Build history of the part. All positions in model axes, mm. Face numbers are marked on the shaded views. Round coordinates to 2 decimals unless told otherwise and drop trailing zeros. One line per item, written item: value. Start each with the question number.
Item 1: Pin check, flat tips, straight feed: pin 1 (3.5 mm diameter, centred on x = 11.5, z = 5, fed in from -Y); pin 2 (4 mm diameter, centred on x = 7.5, z = 0, fed in from -Y); pin 3 (2.5 mm diameter, centred on x = 11.96, z = 11.94, fed in from -Y). Stop position of each tip, or through.
Item 2: Band-saw the part on A-A, the plane y = -2.1. Give the number of separate pieces and of enclosed holes in the cut face, then the cut area to 3 significant figures.
Item 3: Probe L1, parallel to Z at x = -20.5, y = -1.85 (3 decimals); L2, parallel to X at y = -2.75, z = 5.5 (3 decimals); L3, parallel to Z at x = 13, y = -0.75 (3 decimals). List the from-to ranges inside material, lowest first.
Item 4: Two-plate mould, pull along Z, no slides. Class the marked faces 1 and 2: +Z half, -Z half, draft (parallel to the pull), parting line (faces both ways), or undercut.
```python
from build123d import *

# Parameters (mm, degrees)
SKETCH1_W           = 47.81
SKETCH1_H           = 31.85
BOSS_EXTRUDE1_DEPTH = 3.16
SKETCH2_R           = 2.445
BOSS_EXTRUDE2_DEPTH = 1.7
SHELL1_T            = -0.78
SKETCH3_R           = 2.35
SKETCH3_R_2         = 2.175
BOSS_EXTRUDE3_DEPTH = 2.18


with BuildPart() as part:
    # Sketch1 → Boss-Extrude1 (new body)
    with BuildSketch(Plane(origin=(0, 0, 0), x_dir=(1, 0, 0), z_dir=(0, 1, 0))):
        Rectangle(SKETCH1_W, SKETCH1_H)
    extrude(amount=-BOSS_EXTRUDE1_DEPTH)

    # Sketch2 → Boss-Extrude2 (add)
    with BuildSketch(Plane(origin=(0, 0, 0), x_dir=(1, 0, 0), z_dir=(0, 1, 0))):
        with Locations(Location((19.920833333, 11.94375, 0), (0, 0, 270))):
            Circle(SKETCH2_R)
        with Locations(Location((11.960833333, 11.94375, 0), (0, 0, 270))):
            Circle(SKETCH2_R)
        with Locations(Location((4.000833333, 11.94375, 0), (0, 0, 270))):
            Circle(SKETCH2_R)
        with Locations(Location((-3.959166667, 11.94375, 0), (0, 0, 270))):
            Circle(SKETCH2_R)
        with Locations(Location((-11.919166667, 11.94375, 0), (0, 0, 270))):
            Circle(SKETCH2_R)
        with Locations(Location((-19.879166667, 11.94375, 0), (0, 0, 270))):
            Circle(SKETCH2_R)
        with Locations(Location((11.960833333, 3.98375, 0), (0, 0, 270))):
            Circle(SKETCH2_R)
        with Locations(Location((4.000833333, 3.98375, 0), (0, 0, 270))):
            Circle(SKETCH2_R)
        with Locations(Location((-3.959166667, 3.98375, 0), (0, 0, 270))):
            Circle(SKETCH2_R)
        with Locations(Location((-11.919166667, 3.98375, 0), (0, 0, 270))):
            Circle(SKETCH2_R)
        with Locations(Location((-19.879166667, 3.98375, 0), (0, 0, 270))):
            Circle(SKETCH2_R)
        with Locations(Location((11.960833333, -3.97625, 0), (0, 0, 270))):
            Circle(SKETCH2_R)
        with Locations(Location((4.000833333, -3.97625, 0), (0, 0, 270))):
            Circle(SKETCH2_R)
        with Locations(Location((-3.959166667, -3.97625, 0), (0, 0, 270))):
            Circle(SKETCH2_R)
        with Locations(Location((-11.919166667, -3.97625, 0), (0, 0, 270))):
            Circle(SKETCH2_R)
        with Locations(Location((-19.879166667, -3.97625, 0), (0, 0, 270))):
            Circle(SKETCH2_R)
        with Locations(Location((11.960833333, -11.93625, 0), (0, 0, 270))):
            Circle(SKETCH2_R)
        with Locations(Location((4.000833333, -11.93625, 0), (0, 0, 270))):
            Circle(SKETCH2_R)
        with Locations(Location((-3.959166667, -11.93625, 0), (0, 0, 270))):
            Circle(SKETCH2_R)
        with Locations(Location((-11.919166667, -11.93625, 0), (0, 0, 270))):
            Circle(SKETCH2_R)
        with Locations(Location((-19.879166667, -11.93625, 0), (0, 0, 270))):
            Circle(SKETCH2_R)
        with Locations(Location((19.920833333, 3.98375, 0), (0, 0, 270))):
            Circle(SKETCH2_R)
        with Locations(Location((19.920833333, -3.97625, 0), (0, 0, 270))):
            Circle(SKETCH2_R)
        with Locations(Location((19.920833333, -11.93625, 0), (0, 0, 270))):
            Circle(SKETCH2_R)
    extrude(amount=BOSS_EXTRUDE2_DEPTH)

    # Shell1
    shell1_openings = [part.faces().sort_by_distance(p)[0] for p in [
        (0, -3.16, 0),
    ]]
    offset(amount=SHELL1_T, openings=shell1_openings, kind=Kind.INTERSECTION)

    # Sketch3 → Boss-Extrude3 (add)
    # profile 1 of 15: a face of its own
    with BuildSketch(Plane.XZ.offset(0.78)):
        with Locations(Location((-15.936666667, 7.9625, 0), (0, 0, 90))):
            Circle(SKETCH3_R)
        with Locations(Location((-15.936666667, 7.9625, 0), (0, 0, 90))):
            Circle(SKETCH3_R_2, mode=Mode.SUBTRACT)
    # profile 2 of 15: a face of its own
    with BuildSketch(Plane.XZ.offset(0.78)):
        with Locations(Location((-7.966666667, 7.9625, 0), (0, 0, 90))):
            Circle(SKETCH3_R)
        with Locations(Location((-7.966666667, 7.9625, 0), (0, 0, 90))):
            Circle(SKETCH3_R_2, mode=Mode.SUBTRACT)
    # profile 3 of 15: a face of its own
    with BuildSketch(Plane.XZ.offset(0.78)):
        with Locations(Location((0.003333333, 7.9625, 0), (0, 0, 90))):
            Circle(SKETCH3_R)
        with Locations(Location((0.003333333, 7.9625, 0), (0, 0, 90))):
            Circle(SKETCH3_R_2, mode=Mode.SUBTRACT)
    # profile 4 of 15: a face of its own
    with BuildSketch(Plane.XZ.offset(0.78)):
        with Locations(Location((7.973333333, 7.9625, 0), (0, 0, 90))):
            Circle(SKETCH3_R)
        with Locations(Location((7.973333333, 7.9625, 0), (0, 0, 90))):
            Circle(SKETCH3_R_2, mode=Mode.SUBTRACT)
    # profile 5 of 15: a face of its own
    with BuildSketch(Plane.XZ.offset(0.78)):
        with Locations(Location((15.943333333, 7.9625, 0), (0, 0, 90))):
            Circle(SKETCH3_R)
        with Locations(Location((15.943333333, 7.9625, 0), (0, 0, 90))):
            Circle(SKETCH3_R_2, mode=Mode.SUBTRACT)
    # profile 6 of 15: a face of its own
    with BuildSketch(Plane.XZ.offset(0.78)):
        with Locations(Location((-7.966666667, 0.0025, 0), (0, 0, 90))):
            Circle(SKETCH3_R)
        with Locations(Location((-7.966666667, 0.0025, 0), (0, 0, 90))):
            Circle(SKETCH3_R_2, mode=Mode.SUBTRACT)
    # profile 7 of 15: a face of its own
    with BuildSketch(Plane.XZ.offset(0.78)):
        with Locations(Location((0.003333333, 0.0025, 0), (0, 0, 90))):
            Circle(SKETCH3_R)
        with Locations(Location((0.003333333, 0.0025, 0), (0, 0, 90))):
            Circle(SKETCH3_R_2, mode=Mode.SUBTRACT)
    # profile 8 of 15: a face of its own
    with BuildSketch(Plane.XZ.offset(0.78)):
        with Locations(Location((7.973333333, 0.0025, 0), (0, 0, 90))):
            Circle(SKETCH3_R)
        with Locations(Location((7.973333333, 0.0025, 0), (0, 0, 90))):
            Circle(SKETCH3_R_2, mode=Mode.SUBTRACT)
    # profile 9 of 15: a face of its own
    with BuildSketch(Plane.XZ.offset(0.78)):
        with Locations(Location((15.943333333, 0.0025, 0), (0, 0, 90))):
            Circle(SKETCH3_R)
        with Locations(Location((15.943333333, 0.0025, 0), (0, 0, 90))):
            Circle(SKETCH3_R_2, mode=Mode.SUBTRACT)
    # profile 10 of 15: a face of its own
    with BuildSketch(Plane.XZ.offset(0.78)):
        with Locations(Location((-7.966666667, -7.9575, 0), (0, 0, 90))):
            Circle(SKETCH3_R)
        with Locations(Location((-7.966666667, -7.9575, 0), (0, 0, 90))):
            Circle(SKETCH3_R_2, mode=Mode.SUBTRACT)
    # profile 11 of 15: a face of its own
    with BuildSketch(Plane.XZ.offset(0.78)):
        with Locations(Location((0.003333333, -7.9575, 0), (0, 0, 90))):
            Circle(SKETCH3_R)
        with Locations(Location((0.003333333, -7.9575, 0), (0, 0, 90))):
            Circle(SKETCH3_R_2, mode=Mode.SUBTRACT)
    # profile 12 of 15: a face of its own
    with BuildSketch(Plane.XZ.offset(0.78)):
        with Locations(Location((7.973333333, -7.9575, 0), (0, 0, 90))):
            Circle(SKETCH3_R)
        with Locations(Location((7.973333333, -7.9575, 0), (0, 0, 90))):
            Circle(SKETCH3_R_2, mode=Mode.SUBTRACT)
    # profile 13 of 15: a face of its own
    with BuildSketch(Plane.XZ.offset(0.78)):
        with Locations(Location((15.943333333, -7.9575, 0), (0, 0, 90))):
            Circle(SKETCH3_R)
        with Locations(Location((15.943333333, -7.9575, 0), (0, 0, 90))):
            Circle(SKETCH3_R_2, mode=Mode.SUBTRACT)
    # profile 14 of 15: a face of its own
    with BuildSketch(Plane.XZ.offset(0.78)):
        with Locations(Location((-15.936666667, 0.0025, 0), (0, 0, 90))):
            Circle(SKETCH3_R)
        with Locations(Location((-15.936666667, 0.0025, 0), (0, 0, 90))):
            Circle(SKETCH3_R_2, mode=Mode.SUBTRACT)
    # profile 15 of 15: a face of its own
    with BuildSketch(Plane.XZ.offset(0.78)):
        with Locations(Location((-15.936666667, -7.9575, 0), (0, 0, 90))):
            Circle(SKETCH3_R)
        with Locations(Location((-15.936666667, -7.9575, 0), (0, 0, 90))):
            Circle(SKETCH3_R_2, mode=Mode.SUBTRACT)
    extrude(amount=BOSS_EXTRUDE3_DEPTH)


solid = part.part
```
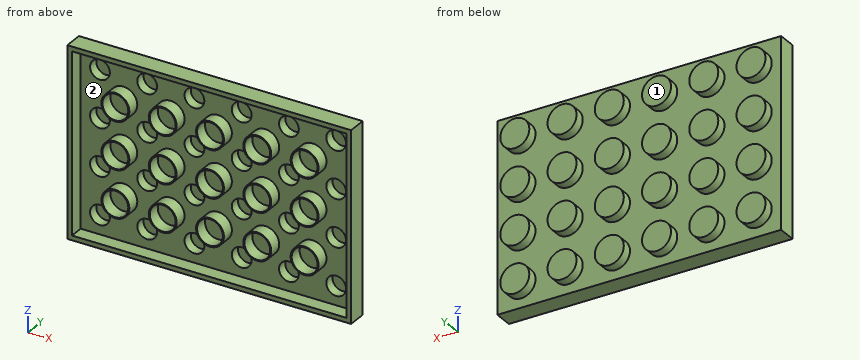
Output:
1. pin 1: stops at y = -0.78
1. pin 2: stops at y = -2.96
1. pin 3: stops at y = 0.92
2. separate pieces: 16
2. enclosed holes: 16
2. area: 159 mm²
3. L1: z = -15.925 to -15.145, 15.145 to 15.925
3. L2: x = -23.905 to -23.125, 23.125 to 23.905
3. L3: z = -15.925 to -13.245, -10.643 to -5.285, -2.683 to 2.675, 5.277 to 10.635, 13.237 to 15.925
4. face 1: draft
4. face 2: undercut
